Check sheet for the modelled part. Datum: model origin and axes. Units: mm. Face numbers are marked on the shaded views. A direction names the side the tool comes from. Give positions to 0.01 mm unless a question says otherwise; leave off trailing zeros. Write each loop counter-clockwise with the first axis right and the second up, starting at its lowest first coordinate (ties: lowest second). Pieces come first, ordered by that corner, then holes. Notation, with made-up numbers: M -13.5,87.25 L 35.5,87.25 A29 cw 35.5,126.25 Z; hole C -6,80.5 d4. An arc over 180 degrees is marked long. Write each question's results on one line, items separated by ' | '. Start each with the question number.
from build123d import *

# Parameters (mm, degrees)
F0_W        = 200
F0_H        = 200
F1_DEPTH    = 40
F3_DEPTH    = 12
F4_DEPTH    = 18
F5_T1_DEPTH = 62.2240943671


# Not quite as in the source:
# - a fillet or chamfer that OpenCascade refuses, or shapes differently, is made with other operations: its cross-section is extruded or revolved along the edge and cut away or added


with BuildPart() as f1:
    # F0 (on Top) → F1 (new body)
    with BuildSketch(Plane.XY):
        with Locations((-2.2933091968, 13.0733736824)):
            Rectangle(F0_W, F0_H)
    extrude(amount=F1_DEPTH)

    # F2 (on face) → F3 (join)
    with BuildSketch(Plane.XY.offset(40)):
        with BuildLine():
            Line((56.2270847505, 13.0733736824), (60.1964650758, 13.0733736824))
            ThreePointArc((60.1964650758, 13.0733736824), (8.8432450397, 74.5627959303), (-60.8137031442, 34.9899286326))
            ThreePointArc((-60.8137031442, 34.9899286326), (-62.7983933068, 24.0316511575), (-60.8137031442, 13.0733736824))
            Line((-60.8137031442, 13.0733736824), (-2.2933091968, 13.0733736824))
            ThreePointArc((-2.2933091968, 13.0733736824), (26.9668877768, 33.3599833436), (56.2270847505, 13.0733736824))
        make_face()
        with BuildLine():
            Line((-2.2933091968, 13.0733736824), (-60.8137031442, 13.0733736824))
            ThreePointArc((-60.8137031442, 13.0733736824), (-31.5535061705, -7.2132359788), (-2.2933091968, 13.0733736824))
        make_face()
        with BuildLine():
            ThreePointArc((-64.7830834694, 13.0733736824), (-13.4298634334, -48.4160485655), (56.2270847505, -8.8431812678))
            ThreePointArc((56.2270847505, -8.8431812678), (58.2117749131, 2.1150962073), (56.2270847505, 13.0733736824))
            Line((56.2270847505, 13.0733736824), (-2.2933091968, 13.0733736824))
            ThreePointArc((-2.2933091968, 13.0733736824), (-31.5535061705, -7.2132359788), (-60.8137031442, 13.0733736824))
            Line((-60.8137031442, 13.0733736824), (-64.7830834694, 13.0733736824))
        make_face()
        with BuildLine():
            ThreePointArc((-60.8137031442, 13.0733736824), (-62.7983933068, 24.0316511575), (-60.8137031442, 34.9899286326))
            ThreePointArc((-60.8137031442, 34.9899286326), (-63.7827314447, 24.2099279189), (-64.7830834694, 13.0733736824))
            Line((-64.7830834694, 13.0733736824), (-60.8137031442, 13.0733736824))
        make_face()
        with BuildLine():
            Line((-2.2933091968, 13.0733736824), (56.2270847505, 13.0733736824))
            ThreePointArc((56.2270847505, 13.0733736824), (26.9668877768, 33.3599833436), (-2.2933091968, 13.0733736824))
        make_face()
        with BuildLine():
            ThreePointArc((56.2270847505, -8.8431812678), (59.196113051, 1.9368194459), (60.1964650758, 13.0733736824))
            Line((60.1964650758, 13.0733736824), (56.2270847505, 13.0733736824))
            ThreePointArc((56.2270847505, 13.0733736824), (58.2117749131, 2.1150962073), (56.2270847505, -8.8431812678))
        make_face()
    extrude(amount=F3_DEPTH)

    # F2 (on face) → F4 (join)
    with BuildSketch(Plane.XY.offset(40)):
        with BuildLine():
            Line((56.2270847505, 13.0733736824), (60.1964650758, 13.0733736824))
            ThreePointArc((60.1964650758, 13.0733736824), (8.8432450397, 74.5627959303), (-60.8137031442, 34.9899286326))
            ThreePointArc((-60.8137031442, 34.9899286326), (-62.7983933068, 24.0316511575), (-60.8137031442, 13.0733736824))
            Line((-60.8137031442, 13.0733736824), (-2.2933091968, 13.0733736824))
            ThreePointArc((-2.2933091968, 13.0733736824), (26.9668877768, 33.3599833436), (56.2270847505, 13.0733736824))
        make_face()
        with BuildLine():
            Line((-2.2933091968, 13.0733736824), (-60.8137031442, 13.0733736824))
            ThreePointArc((-60.8137031442, 13.0733736824), (-31.5535061705, -7.2132359788), (-2.2933091968, 13.0733736824))
        make_face()
        with BuildLine():
            ThreePointArc((56.2270847505, -8.8431812678), (59.196113051, 1.9368194459), (60.1964650758, 13.0733736824))
            Line((60.1964650758, 13.0733736824), (56.2270847505, 13.0733736824))
            ThreePointArc((56.2270847505, 13.0733736824), (58.2117749131, 2.1150962073), (56.2270847505, -8.8431812678))
        make_face()
    extrude(amount=F4_DEPTH)

    # F5: fillet of radius 1.96 on 2 edges, made by hand

    # F5_s2 → F5_t1 (cut)
    with BuildSketch(Plane.XY.offset(52)):
        with BuildLine():
            ThreePointArc((60.196077506, 13.2934603584), (58.5741142709, 11.3559254547), (56.3903482373, 12.627134387))
            ThreePointArc((56.3903482373, 12.627134387), (58.2108716144, 1.8775122879), (56.2270847505, -8.8431812678))
            ThreePointArc((56.2270847505, -8.8431812678), (59.2156290063, 2.0451186179), (60.196077506, 13.2934603584))
        make_face()
    extrude(amount=F5_T1_DEPTH, mode=Mode.SUBTRACT)


solid = f1.part
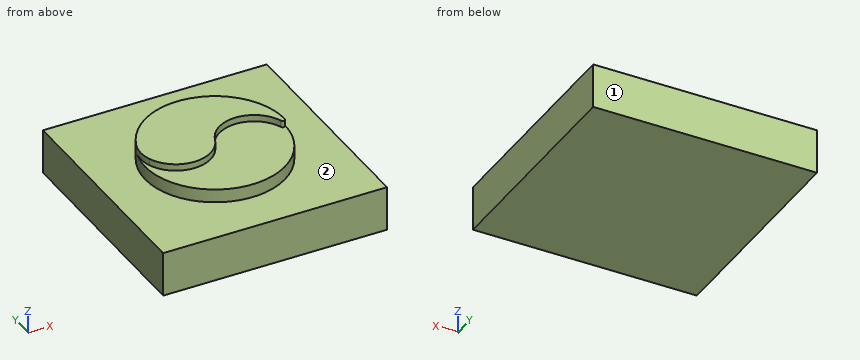
Q1. Section check D-D on x = -40.5. Record the boundary of the cut face in (y, z) (3 decimals), plus the area to 3 significant figures.
Q2. Tool access check on the marked faces 1 and 2. Record the directions out of +Z, -Z, +X, -X, +Y, -Y that give a thin tool (end or side, any length) a straight path to the whole face; none if there is none.
Q3. Scan lines: L1, parallel to Z at x = -61, y = 96; L2, parallel to Z at x = 25.5, y = 12.5; L3, parallel to Y at x = 32.5, z = 51. Record each from-to range of solid material in increasing order.
Q4. Depth check by flat-ended pin: pin 1 Ø10 at (y, z) = (36, 50) entering from -X; pin 2 Ø5 at (x, y) = (7.5, -43) entering from +Z; pin 3 Ø5 at (x, y) = (48, -43) entering from +Z. Enter the tip coordinate at first touch or a pass-through.
Q5. Section check A-A on y = 57. Record the boundary of the cut face in (x, z), plus the area to 3 significant figures.
Q6. Section check C-C on z = 44. Record the boundary of the cut face in (x, y), plus the area to 3 significant figures.
Q7. Section check B-B on x = 48.5. Record the boundary of the cut face in (y, z), plus the area to 3 significant figures.
Check result:
1) outline: M -86.927,0 L 113.073,0 L 113.073,40 L 62.523,40 L 62.523,58 L -5.905,58 L -5.905,52 L -36.376,52 L -36.376,40 L -86.927,40 Z | area: 9,600 mm^2
2) face 1: +Z, -Z, +X, -X, +Y | face 2: +Z
3) L1: 0 to 40 | L2: 0 to 52 | L3: -38.83 to 64.98
4) pin 1: x = -62.16 | pin 2: z = 52 | pin 3: z = 40
5) outline: M -102.29,0 L 97.71,0 L 97.71,40 L 42.15,40 L 42.15,58 L -46.74,58 L -46.74,40 L -102.29,40 Z | area: 9,600 mm^2
6) outline: C -2.29,13.07 d124.98 | area: 12,300 mm^2
7) outline: M -86.93,0 L 113.07,0 L 113.07,40 L 49.47,40 L 49.47,58 L 24.76,58 L 24.76,52 L -23.33,52 L -23.33,40 L -86.93,40 Z | area: 9,020 mm^2
